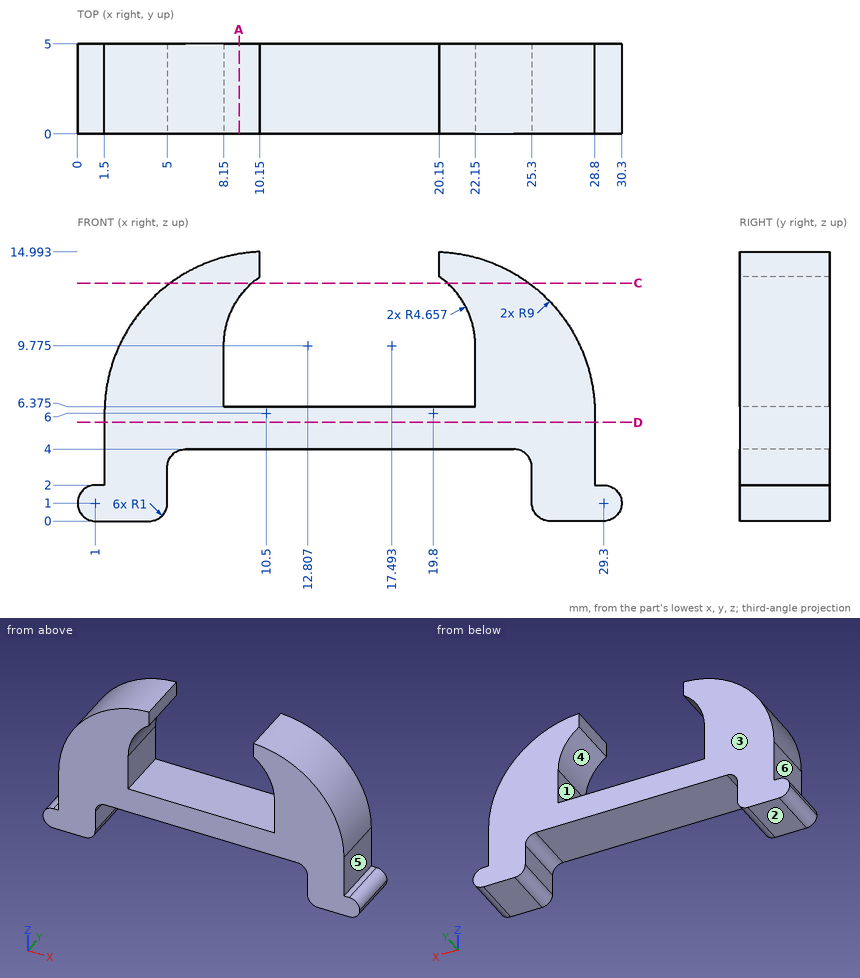
Can you work these out from the drawing? Everything is in mm from the part's minimum corner. A direction names the side the tool comes from. Give positions to 0.01 mm unless a question says otherwise; leave off trailing zeros. Order: outer loops, then holes, each group sorted by start corner. A loop starts at its lowest first (then second) coordinate and runs counter-clockwise, first axis right, second up. Notation, with made-up numbers: M 67.25,39 L 83.25,39 A27 ccw 83.25,60 Z; hole C 3.5,65 d7. An arc over 180 degrees is marked long. Use a Markdown table: item, result. Add a question column.
Item 1: Suppose I cut it at C-C (z = 13.25). List the corners of the cut face in (x, y) for me.
Item 2: If I drill on L1, parallel to Z at x = 12.5, y = 3.3 (1 decimal); L2, parallel to X at y = 0.6, z = 9.5; L3, parallel to Z at x = 10, y = 0.5 (1 decimal), over which ranges is the centre line in solid material (lowest first)? Write a range as [from, to].
Item 3: Will these pins go through, and if not, where does the flat tip stop? pin 1 (1.7 mm diameter, centred on y = 1.5, z = 7, fed in from -X); pin 2 (2 mm diameter, centred on y = 1.5, z = 5, fed in from +X); pin 3 (2.5 mm diameter, centred on x = 12, y = 2, fed in from +Z) (3 decimals).
Item 4: We'd pull the mould along Z, two halves only. Please class the marked faces 1, 2 and 3: +Z half, -Z half, draft (parallel to the pull), parting line (faces both ways), or undercut.
Item 5: For the marked faces 4, 5 and 6, which set-ups out of +Z, -Z, +X, -X, +Y, -Y let a thin tool reach every point of the face, with its end or its side?
Item 6: Suppose I cut it at A-A (x = 9). List the corners of the cut face in (y, z) for me (1 decimal).
Item 7: Suppose I cut it at D-D (z = 5.5). List the corners of the cut face in (x, y) for me.
Answer sheet:
| question | item | result |
|---|---|---|
| 1 | outline | M 5.17,0 L 9.71,0 L 9.71,5 L 5.17,5 Z; M 20.59,0 L 25.13,0 L 25.13,5 L 20.59,5 Z |
| 2 | L1 | z = [4, 6.4] |
| 2 | L2 | x = [2.21, 8.15], [22.15, 28.09] |
| 2 | L3 | z = [4, 6.4], [13.5, 15] |
| 3 | pin 1 | stops at x = 1.5 |
| 3 | pin 2 | stops at x = 28.8 |
| 3 | pin 3 | stops at z = 6.375 |
| 4 | face 1 | undercut |
| 4 | face 2 | -Z half |
| 4 | face 3 | draft |
| 5 | face 4 | +Y, -Y |
| 5 | face 5 | +Z, +X, +Y, -Y |
| 5 | face 6 | +Z, -X, +Y, -Y |
| 6 | outline | M 0,4 L 5,4 L 5,6.4 L 0,6.4 Z; M 0,12.5 L 5,12.5 L 5,14.9 L 0,14.9 Z |
| 7 | outline | M 1.5,0 L 28.8,0 L 28.8,5 L 1.5,5 Z |
